Can you work these out from the model? Positions are in its coordinate system, mm. Face numbers are marked on the shaded views. A direction names the side the tool comes from. Coordinates: 2 decimals unless noted, no trailing zeros. Order: outer loops, then holes, each group sorted by start corner. A loop starts at its lowest first (then second) coordinate and runs counter-clockwise, first axis right, second up. Notation, with made-up numbers: (0.25, 62) -> (33.25, 62) arc R16 cw to (33.25, 69) -> close; hole circle Ø11 at (31.25, 85.5). An arc over 180 degrees is marked (long way). Write item = value, one per line.
```python
from build123d import *

# Parameters (mm, degrees)
SALIENTE_EXTRUIR1_DEPTH = 14
REDONDEO1_R             = 3
CROQUIS2_R              = 2.5
CORTAR_EXTRUIR1_DEPTH   = 10


with BuildPart() as part:
    # Croquis1 → Saliente-Extruir1 (new body)
    with BuildSketch(Plane(origin=(0, 0, 0), x_dir=(1, 0, 0), z_dir=(0, 1, 0))):
        with BuildLine():
            Line((-20, 0), (-8, 0))
            Line((-8, 0), (-8, 8))
            ThreePointArc((-8, 8), (0, 16), (8, 8))
            Line((8, 8), (8, 0))
            Line((8, 0), (20, 0))
            Line((20, 0), (20, 1))
            Line((20, 1), (9, 1))
            Line((9, 1), (9, 8))
            ThreePointArc((9, 8), (0, 17), (-9, 8))
            Line((-9, 8), (-8.998859232, 7.856708279))
            Line((-8.998859232, 7.856708279), (-8.94427191, 1))
            Line((-8.94427191, 1), (-20, 1))
            Line((-20, 1), (-20, 0))
        make_face()
    extrude(amount=SALIENTE_EXTRUIR1_DEPTH)

    # Redondeo1
    redondeo1_edges = [part.edges().sort_by_distance(p)[0] for p in [
        (-20, 0, -0.5),
        (20, 0, -0.5),
        (20, 14, -0.5),
        (-20, 14, -0.5),
    ]]
    fillet(redondeo1_edges, radius=REDONDEO1_R)

    # Croquis2 → Cortar-Extruir1 (cut)
    with BuildSketch(Plane.XY):
        with Locations((-16.5, 6.5)):
            Circle(CROQUIS2_R)
        with Locations((16.5, 6.5)):
            Circle(CROQUIS2_R)
    extrude(amount=-CORTAR_EXTRUIR1_DEPTH, mode=Mode.SUBTRACT)


solid = part.part
```
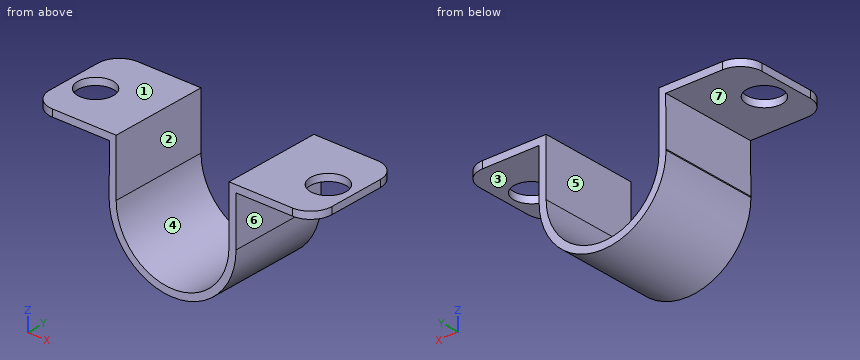
Item 1: I'm going to push flat-ended pins straight in: P1, Ø4, axis at x = 11, z = -9.5, coming from the +Y side; P2, Ø4, axis at x = 12, y = 12, coming from the -Z side; P3, Ø3, axis at x = 0.5, y = 4, coming from the +Z side; P4, Ø5.5, axis at y = 9.5, z = -4, coming from the +X side. Where does each tip first touch, or does it pass through?
A:
P1 = through
P2 = -1
P3 = -15.75
P4 = 9
Item 2: I want a section at A-A, the plane y = 8. Please give me the cut outline in (x, z), plus the area to 3 significant figures.
A:
outline = (-20, -1) -> (-18.5, -1) -> (-18.5, 0) -> (-20, 0) -> close; (-14.5, -1) -> (-8.94, -1) -> (-9, -8) arc R9 ccw to (9, -8) -> (9, -1) -> (14.5, -1) -> (14.5, 0) -> (8, 0) -> (8, -8) arc R8 cw to (-8, -8) -> (-8, 0) -> (-14.5, 0) -> close; (18.5, -1) -> (20, -1) -> (20, 0) -> (18.5, 0) -> close
area = 56.5 mm2
Item 3: I want a section at D-D, the plane y = 4.5. Please give me the cut outline in (x, z), plus the area to 3 significant figures.
A:
outline = (-20, -1) -> (-18, -1) -> (-18, 0) -> (-20, 0) -> close; (-15, -1) -> (-8.94, -1) -> (-9, -8) arc R9 ccw to (9, -8) -> (9, -1) -> (15, -1) -> (15, 0) -> (8, 0) -> (8, -8) arc R8 cw to (-8, -8) -> (-8, 0) -> (-15, 0) -> close; (18, -1) -> (20, -1) -> (20, 0) -> (18, 0) -> close
area = 58.5 mm2
Item 4: If we mould it in two halves opening along X, with no side actions, what happens to the marked faces 4, 5, 6 and 7? For each: pulls with the +X half, pulls with the -X half, needs draft (parallel to the pull), parting line crosses it, or undercut.
A:
face_4 = undercut
face_5 = undercut
face_6 = pulls with the +X half
face_7 = needs draft
Item 5: I want a section at B-B, the plane x = -16.5. Please give me the cut outline in (y, z), plus the area to 3 significant figures.
A:
outline = (0, -1) -> (4, -1) -> (4, 0) -> (0, 0) -> close; (9, -1) -> (14, -1) -> (14, 0) -> (9, 0) -> close
area = 9.00 mm2
Item 6: I want a section at C-C, the plane z = -14. Please give me the cut outline in (x, y), plus the area to 3 significant figures.
A:
outline = (-6.71, 0) -> (-5.29, 0) -> (-5.29, 14) -> (-6.71, 14) -> close; (5.29, 0) -> (6.71, 0) -> (6.71, 14) -> (5.29, 14) -> close
area = 39.7 mm2
Item 7: For the marked faces 1, 2 and 3, which set-ups out of +Z, -Z, +X, -X, +Y, -Y let a thin tool reach every point of the face, with its end or its side?
A:
face_1 = +Z, +X, -X, +Y, -Y
face_2 = +Z, +Y, -Y
face_3 = -Z, +X, +Y, -Y
Item 8: If I drill on probe 1 along Y at (x, z) = (16.5, -0.6); probe 2 along X at (y, z) = (7.75, -11.25); probe 3 along Z at (x, y) = (-17, 12.25), over which ranges is the centre line in solid material (lowest first)?
A:
probe_1 = 0 to 4, 9 to 14
probe_2 = -8.39 to -7.31, 7.31 to 8.39
probe_3 = -1 to 0
